Source: three-view drawing plus pictorial views. Frame: mm from the lowest corner of the part. A direction names the side the tool comes from. Give positions to 0.01 mm unless a question says otherwise; leave off trailing zeros. Loops run counter-clockwise (first coordinate to the right, second up) from the corner with the lowest first, then second, coordinate; pieces in that order, holes last. Notation, with made-up numbers: M -15.75,43 L 37.25,43 A26 cw 37.25,77 Z; hole C -38,-29 d2. An arc over 180 degrees is marked long. Answer as a JSON object with one key per item and string values. Group by question number.
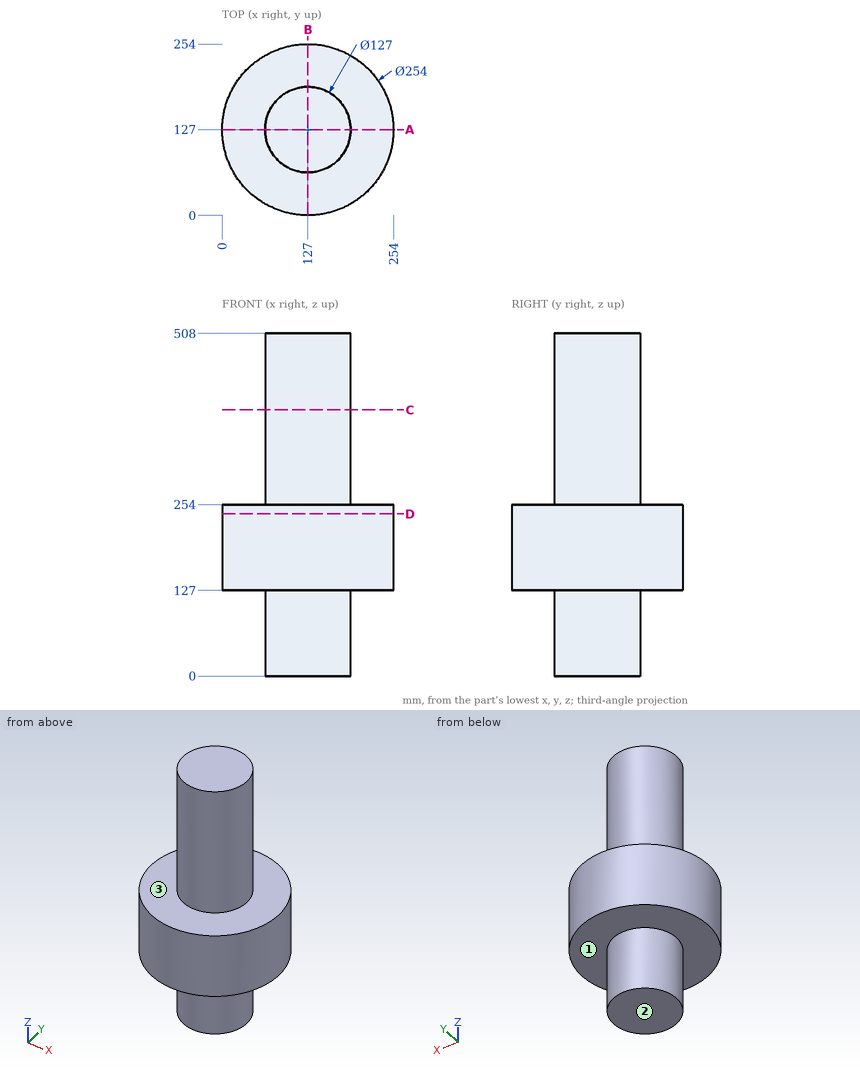
1. Section D-D (z = 240.5). Output: boundary loops of the cut face in (x, y), then the cut area to 3 significant figures.
2. Section C-C (z = 394.5). Output: boundary loops of the cut face in (x, y).
3. Material intervals for L1, parallel to Z at x = 25, y = 175.5; L2, parallel to Y at x = 128.5, z = 334; L3, parallel to Y at x = 124.5, z = 452, sorted ascending.
4. First-contact query: P1, Ø8, axis at y = 197.5, z = 157, coming from the +X side; P2, Ø1.5, axis at y = 179.5, z = 58, coming from the +X side; P3, Ø6, axis at y = 163, z = 418.5, coming from the -X side. Flat tips, straight axial feed; report the tip coordinate or a pass-through.
5. Section A-A (y = 127). Output: boundary loops of the cut face in (x, z), then the cut area to 3 significant figures.
6. Reachability of the marked faces 1, 2 and 3 from +Z, -Z, +X, -X, +Y, -Y: full face, straight path, thin tool, end or side. Return the list, or none.
Geometry results:
{
 "1": {"outline": "C 127,127 d254", "area": "50,700 mm2"},
 "2": {"outline": "C 127,127 d127"},
 "3": {"L1": "127 to 254", "L2": "63.52 to 190.48", "L3": "63.55 to 190.45"},
 "4": {"P1": "x = 235.2", "P2": "x = 163.8", "P3": "x = 72.75"},
 "5": {"outline": "M 0,127 L 63.5,127 L 63.5,0 L 190.5,0 L 190.5,127 L 254,127 L 254,254 L 190.5,254 L 190.5,508 L 63.5,508 L 63.5,254 L 0,254 Z", "area": "80,600 mm2"},
 "6": {"face 1": "-Z", "face 2": "-Z, +X, -X, +Y, -Y", "face 3": "+Z"}
}
